from build123d import *

# Parameters (mm, degrees)
PAD013_DEPTH    = 5
SKETCH029_R     = 1.8
POCKET014_DEPTH = 2
POCKET015_DEPTH = 3.2
SKETCH031_R     = 1.8
POCKET016_DEPTH = 21.859536
CHAMFER004_SIZE = 1


with BuildPart() as part:
    # Sketch028 → Pad013 (new body, symmetric)
    with BuildSketch(Plane.YZ):
        with BuildLine():
            Line((94, -15), (76, -15))
            Line((76, -15), (7.068758, -40.08892))
            Line((7.068758, -40.08892), (7.416055, -42.058536))
            Line((7.416055, -42.058536), (86.145177, -24.767201))
            ThreePointArc((86.145177, -24.767201), (91.792682, -21.266906), (94, -15))
        make_face()
    extrude(amount=PAD013_DEPTH, both=True)

    # Sketch029 (on Face1 of Pad013) → Pocket014 (cut)
    with BuildSketch(Plane(origin=(0, 0, -15), x_dir=(0, -1, 0), z_dir=(0, 0, 1))):
        with Locations((-83.35, 0)):
            Circle(SKETCH029_R)
    extrude(amount=-POCKET014_DEPTH, mode=Mode.SUBTRACT)

    # Sketch030 (on Face9 of Pocket014) → Pocket015 (cut)
    with BuildSketch(Plane(origin=(0, 0, -17), x_dir=(0, -1, 0), z_dir=(0, 0, 1))):
        Polygon((-86.35, 1.732051), (-86.35, -1.732051), (-83.35, -3.464102), (-80.35, -1.732051), (-80.35, 1.732051), (-80.35, 3.464102), (-86.35, 3.464102), align=None)
    extrude(amount=-POCKET015_DEPTH, mode=Mode.SUBTRACT)

    # Sketch031 (on Face15 of Pocket015) → Pocket016 (cut, through all)
    with BuildSketch(Plane(origin=(0, 0, -20.2), x_dir=(0, -1, 0), z_dir=(0, 0, 1))):
        with Locations((-83.35, 0)):
            Circle(SKETCH031_R)
    extrude(amount=-POCKET016_DEPTH, mode=Mode.SUBTRACT)

    # Chamfer004
    chamfer004_edges = [part.edges().sort_by_distance(p)[0] for p in [
        (5, 91.792682, -21.266906),
        (-5, 91.792682, -21.266906),
    ]]
    chamfer(chamfer004_edges, length=CHAMFER004_SIZE)


solid = part.part
Here's how the part is built. I have some questions about the finished solid (model axes, mm). A direction names the side the tool comes from. Give positions to 0.01 mm unless a question says otherwise; leave off trailing zeros. Order: outer loops, then holes, each group sorted by start corner. A loop starts at its lowest first (then second) coordinate and runs counter-clockwise, first axis right, second up. Notation, with made-up numbers: M 6,61 L 23,61 A5 cw 23,66 Z; hole C 34,-33.5 d4. An arc over 180 degrees is marked long. Answer as a JSON object with one key per item and string values. Group by question number.
1) Suppose I cut it at B-B, the plane y = 31. Write out the boundary of the cut face in (x, z).
2) On a 3-axis mill with a long thin cutter (end or side, diameter ignored), from which of +Z, -Z, +X, -X, +Y, -Y can I reach the whole of each face in a straight line? I mean faces 1 (the flat face through (2, 82, -17)), 2 (the flat face through (5, 59, -25)). Say none if no direction works.
3) We'd pull the mould along X, two halves only. Please class faces 3 (the cylindrical face through (-0.689, 81.687, -22.949)), 4 (the flat face through (0.07, 7.24, -41.06)), 5 (the flat face through (4.507, 46.121, -33.039)): pulls with the +X half, pulls with the -X half, needs draft (parallel to the pull), parting line crosses it, or undercut.
4) I'm going to push flat-ended pins straight in: pin 1 Ø4 at (x, y) = (0, 83.35) entering from -Z; pin 2 Ø3.5 at (x, z) = (0.5, -18.5) entering from +Y; pin 3 Ø4 at (x, z) = (0, -20) entering from +Y; pin 4 Ø12 at (y, z) = (37, -20) entering from -X. Where does each tip first touch, or does it pass through?
5) Please list where these lines run through material, in increasing order: L1, parallel to X at y = 83.35, z = -23.3; L2, parallel to Z at x = -4.5, y = 73; L3, parallel to Z at x = 4.5, y = 81.5. Write a range as [from, to].
6) Suppose I cut it at A-A, the plane x = 0. Write out the boundary of the cut face in (y, z).
7) Suppose I cut it at C-C, the plane z = -29. Write out the boundary of the cut face in (x, y), plus the area to 3 significant figures.
Results found:
{
 "1": {"outline": "M -5,-35.85 L -4,-36.88 L 4,-36.88 L 5,-35.85 L 5,-31.38 L -5,-31.38 Z"},
 "2": {"face 1": "none", "face 2": "+Z, -Z, +X, +Y, -Y"},
 "3": {"face 3": "undercut", "face 4": "needs draft", "face 5": "pulls with the +X half"},
 "4": {"pin 1": "z = -25.82", "pin 2": "y = 93.85", "pin 3": "y = 93.54", "pin 4": "through"},
 "5": {"L1": "[-5, -1.8], [1.8, 5]", "L2": "[-27.14, -16.09]", "L3": "[-25.28, -15]"},
 "6": {"outline": "M 7.07,-40.09 L 7.42,-42.06 L 81.55,-25.78 L 81.55,-20.2 L 80.35,-20.2 L 80.35,-17 L 81.55,-17 L 81.55,-15 L 76,-15 Z; M 85.15,-24.99 L 86.15,-24.77 A10 ccw 94,-15 L 85.15,-15 L 85.15,-17 L 86.35,-17 L 86.35,-20.2 L 85.15,-20.2 Z"},
 "7": {"outline": "M -5,37.54 L 5,37.54 L 5,62.21 L 4,66.87 L -4,66.87 L -5,62.21 Z", "area": "289 mm²"}
}
